CAD build for the part. Positions are in the model's coordinates, mm. Give positions to 0.01 mm unless a question says otherwise; leave off trailing zeros. Write each loop counter-clockwise with the first axis right and the second up, starting at its lowest first coordinate (ties: lowest second). Pieces come first, ordered by that corner, then holes. Notation, with made-up numbers: (82.5, 32) -> (103.5, 32) arc R15 cw to (103.5, 44) -> close; hole circle Ø6 at (20.5, 3). An arc over 180 degrees is marked (long way). Answer as a JSON object with one key per item and string values.
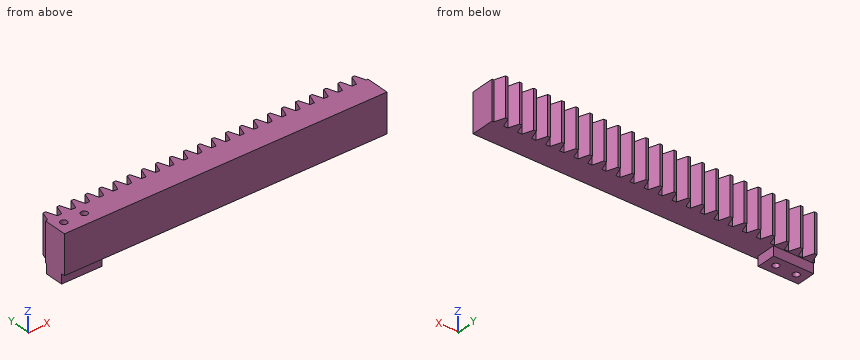
```python
from build123d import *

# Parameters (mm, degrees)
CROQUIS1_W              = 199.517
CROQUIS1_H              = 15.875
SALIENTE_EXTRUIR1_DEPTH = 18.445999938
CORTAR_EXTRUIR3_DEPTH   = 102.759604668
MATRIZL1_COUNT          = 32
MATRIZL1_PITCH          = 6.649704506
CROQUIS5_W              = 19.05
CROQUIS5_H              = 8.992
SALIENTE_EXTRUIR2_DEPTH = 23.00199997
CROQUIS6_R              = 1.5875
CORTAR_EXTRUIR4_DEPTH   = 103.683271428
ESCALA1_SCALE           = 0.25
CROQUIS7_R              = 4.213965504
CORTAR_EXTRUIR5_DEPTH   = 11.684
CROQUIS8_W              = 38.19525
CROQUIS8_H              = 4.611499984
SALIENTE_EXTRUIR3_DEPTH = 0.03


with BuildPart() as part:
    # Croquis1 → Saliente-Extruir1 (new body)
    with BuildSketch(Plane.XY):
        Rectangle(CROQUIS1_W, CROQUIS1_H)
    extrude(amount=SALIENTE_EXTRUIR1_DEPTH)

    # Croquis4 → Cortar-Extruir3 (cut, through all)
    with BuildSketch(Plane.XY.offset(18.445999938)):
        Polygon((-98.7425, 3.1115), (-100.7745, 3.1115), (-102.4636, 7.9375), (-97.0534, 7.9375), align=None)
    cortar_extruir3 = extrude(amount=-CORTAR_EXTRUIR3_DEPTH, mode=Mode.SUBTRACT)

    # MatrizL1: Cortar-Extruir3 ×32
    with Locations(*[(i * MATRIZL1_PITCH, 0, 0) for i in range(1, MATRIZL1_COUNT)]):
        add(cortar_extruir3, mode=Mode.SUBTRACT)

    # Croquis5 → Saliente-Extruir2 (add)
    with BuildSketch(Plane.XY.offset(18.445999938)):
        with Locations((-90.2335, -1.8415)):
            Rectangle(CROQUIS5_W, CROQUIS5_H)
    extrude(amount=-SALIENTE_EXTRUIR2_DEPTH)

    # Croquis6 → Cortar-Extruir4 (cut, through all)
    with BuildSketch(Plane(origin=(0, 0, -4.556000032), x_dir=(-1, 0, 0), z_dir=(0, 0, -1))):
        with Locations((85.4075, -1.8415)):
            Circle(CROQUIS6_R)
        with Locations(Location((95.0595, -1.8415, 0), (0, 0, 180))):
            Circle(CROQUIS6_R)
    extrude(amount=-CORTAR_EXTRUIR4_DEPTH, mode=Mode.SUBTRACT)


with BuildPart() as part_1:
    # Escala1: scaled about (-0.770061652, -1.212816099, 9.056417428)
    add(part.part.scale(ESCALA1_SCALE).moved(Location((-0.577546239, -0.909612074, 6.792313071))))

    # Croquis7 → Cortar-Extruir5 (cut)
    with BuildSketch(Plane(origin=(24.362078761, 0, 0), x_dir=(0, 0, -1), z_dir=(1, 0, 0))):
        with Locations((-9.112278758, -1.455704097)):
            Circle(CROQUIS7_R)
    extrude(amount=-CORTAR_EXTRUIR5_DEPTH, mode=Mode.SUBTRACT)

    # Croquis8 → Saliente-Extruir3 (add)
    with BuildSketch(Plane.XZ.offset(2.893987074)):
        with Locations((-6.419546239, 9.098063063)):
            Rectangle(CROQUIS8_W, CROQUIS8_H)
    extrude(amount=SALIENTE_EXTRUIR3_DEPTH)


solid = part_1.part
```
1) Wall check: probe 1 along X at (y, z) = (-1.45, 9.15); probe 2 along Y at (x, z) = (-22, 10.3); probe 3 along Z at (x, y) = (-2, -0.35). Give the ranges that are in metal, low to high.
Model answer:
{"probe 1": "x = -25.52 to -24.73, -23.95 to -22.32, -21.54 to 12.68", "probe 2": "y = -2.92 to -1.76, -0.98 to -0.13", "probe 3": "z = 6.79 to 11.4"}
2) Slice it at B-B (z = 10.8). State how many separate pieces and enclosed holes the cut face has, then the cut area to 3 significant figures.
Model answer:
{"separate pieces": "1", "enclosed holes": "2", "area": "126 mm2"}
3) Pin check, flat tips, straight feed: pin 1 (1 mm diameter, centred on x = -17.5, z = 8, fed in from +Y); pin 2 (2 mm diameter, centred on x = 6, y = 0, fed in from -Z). Stop position of each tip, or through.
Model answer:
{"pin 1": "stops at y = 1.07", "pin 2": "stops at z = 6.79"}
4) Slice it at A-A (y = -0.6). List the corners of the cut face in (x, z), then the cut area to 3 significant figures.
Model answer:
{"outline": "(-25.52, 5.65) -> (-20.75, 5.65) -> (-20.75, 6.79) -> (12.68, 6.79) -> (12.68, 11.4) -> (-25.52, 11.4) -> close", "area": "182 mm2"}
